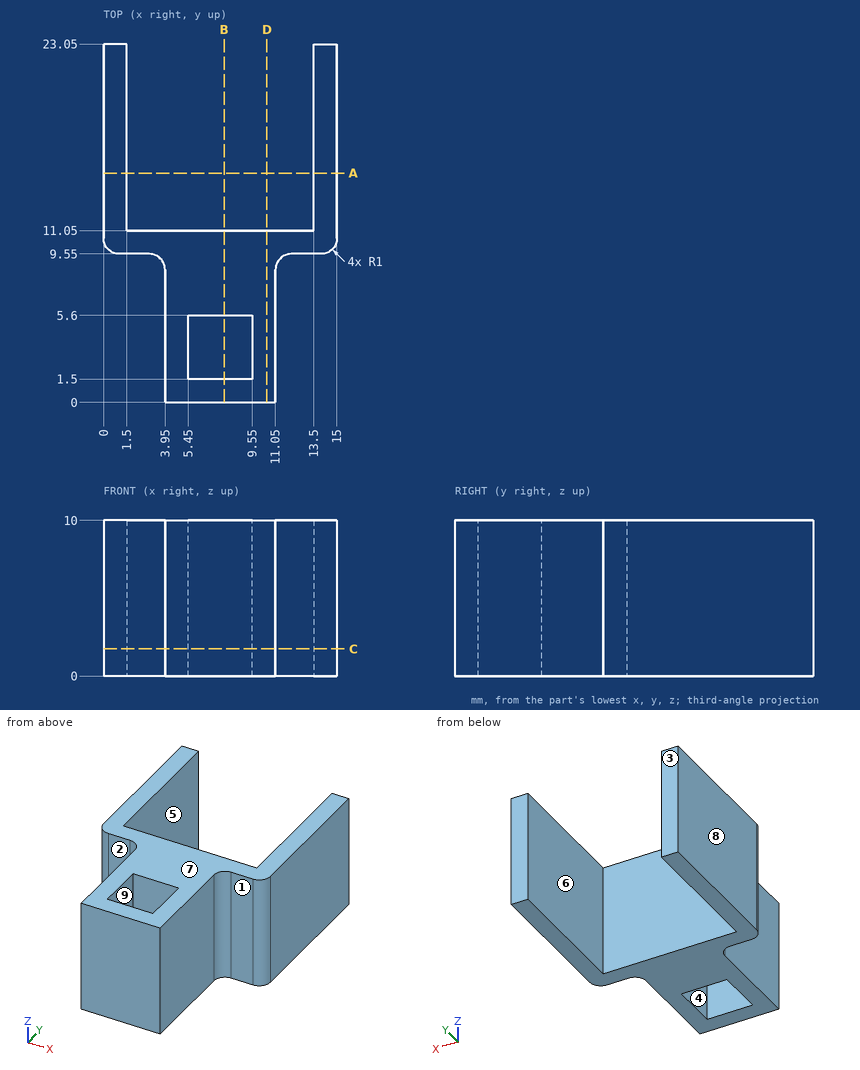
For this review, use the dimensioned drawing (mm, ordinates from the lowest corner) and the shaded views. A direction names the side the tool comes from. Coordinates: 2 decimals unless noted, no trailing zeros. Loops run counter-clockwise (first coordinate to the right, second up) from the corner with the lowest first, then second, coordinate; pieces in that order, holes last. Notation, with made-up numbers: (36, 61) -> (58, 61) arc R17 ccw to (58, 87) -> close; hole circle Ø7 at (3, -33.5). An arc over 180 degrees is marked (long way). Use a Markdown table: item, result. Add a question column.
1. Add section B-B on x = 7.75. Write out the cut boundary in (y, z).
2. Add section A-A on y = 14.75. Write out the cut boundary in (x, z).
3. To check wall thickness, follow line 1 (X direction, y = 14.25, z = 4.5); line 2 (Y direction, x = 7, z = 3.25); line 3 (X direction, y = 6.75, z = 7.5). State the ranges of each line that lie inside material, in increasing order.
4. Draft analysis for pull direction X (two halves, no side actions). For the marked faces 6, 7, 8 and 9, state which applies: pulls with the +X half, pulls with the -X half, needs draft (parallel to the pull), parting line crosses it, or undercut.
5. Add section D-D on x = 10.5. Write out the cut boundary in (y, z).
6. Machinability: for the marked faces 1, 2, 3, 4 and 5, which of the approach directions +Z, -Z, +X, -X, +Y, -Y give a long, thin tool a straight path to every point of the face, cutting with its end or side? Answer none if there is none.
7. Add section C-C on z = 1.75. Write out the cut boundary in (x, y).
8. Clearance check with flat-ended pins moving along their axes: pin 1 Ø2 at (y, z) = (3, 4.5) entering from +X; pin 2 Ø1 at (x, z) = (2, 3) entering from -Y; pin 3 Ø2 at (y, z) = (3, 6) entering from -X; pin 4 Ø2 at (x, y) = (3.5, 13.5) entering from +Z. State where each tip first meets the part, or that it passes through.
Returned:
| question | item | result |
|---|---|---|
| 1 | outline | (0, 0) -> (1.5, 0) -> (1.5, 10) -> (0, 10) -> close; (5.6, 0) -> (11.05, 0) -> (11.05, 10) -> (5.6, 10) -> close |
| 2 | outline | (0, 0) -> (1.5, 0) -> (1.5, 10) -> (0, 10) -> close; (13.5, 0) -> (15, 0) -> (15, 10) -> (13.5, 10) -> close |
| 3 | line 1 | x = 0 to 1.5, 13.5 to 15 |
| 3 | line 2 | y = 0 to 1.5, 5.6 to 11.05 |
| 3 | line 3 | x = 3.95 to 11.05 |
| 4 | face 6 | undercut |
| 4 | face 7 | needs draft |
| 4 | face 8 | pulls with the -X half |
| 4 | face 9 | undercut |
| 5 | outline | (0, 0) -> (11.05, 0) -> (11.05, 10) -> (0, 10) -> close |
| 6 | face 1 | +Z, -Z, +X, -Y |
| 6 | face 2 | +Z, -Z, -X, -Y |
| 6 | face 3 | +Z, -Z, +X, -X, +Y |
| 6 | face 4 | +Z, -Z |
| 6 | face 5 | +Z, -Z, +Y |
| 7 | outline | (0, 10.55) arc R1 ccw to (1, 9.55) -> (2.95, 9.55) arc R1 cw to (3.95, 8.55) -> (3.95, 0) -> (11.05, 0) -> (11.05, 8.55) arc R1 cw to (12.05, 9.55) -> (14, 9.55) arc R1 ccw to (15, 10.55) -> (15, 23.05) -> (13.5, 23.05) -> (13.5, 11.05) -> (1.5, 11.05) -> (1.5, 23.05) -> (0, 23.05) -> close; hole (5.45, 1.5) -> (9.55, 1.5) -> (9.55, 5.6) -> (5.45, 5.6) -> close |
| 8 | pin 1 | stops at x = 11.05 |
| 8 | pin 2 | stops at y = 9.55 |
| 8 | pin 3 | stops at x = 3.95 |
| 8 | pin 4 | passes through |
